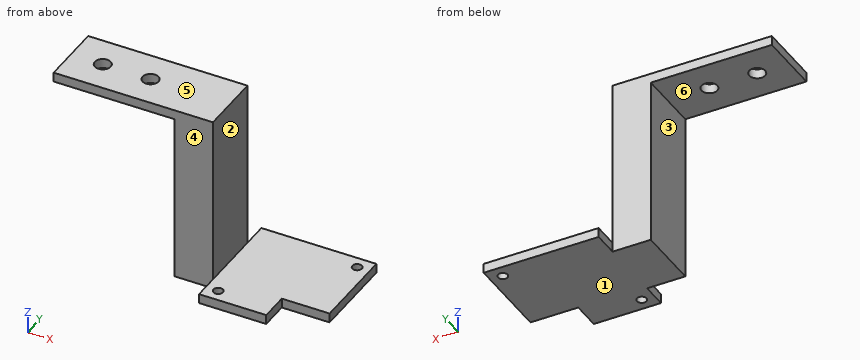
from build123d import *

# Parameters (mm, degrees)
SKETCH_1_W          = 36.1
SKETCH_1_H          = 36.1
EXTRUDE_1_DEPTH     = 3
SKETCH_2_R          = 1.5
CUT_EXTRUDE_1_DEPTH = 3
SKETCH_3_W          = 15
SKETCH_3_H          = 9
CUT_EXTRUDE_2_DEPTH = 3
SKETCH_4_W          = 12
SKETCH_4_H          = 10
EXTRUDE_2_DEPTH     = 3
SKETCH_5_W          = 12
SKETCH_5_H          = 20
EXTRUDE_3_DEPTH     = 50
SKETCH_7_W          = 50
SKETCH_7_H          = 20
EXTRUDE_4_DEPTH     = 3
SKETCH_9_R          = 2.5
CUT_EXTRUDE_4_DEPTH = 3


with BuildPart() as part:
    # 草图1 → 凸台-拉伸1 (new body)
    with BuildSketch(Plane.XY):
        Rectangle(SKETCH_1_W, SKETCH_1_H)
    extrude(amount=EXTRUDE_1_DEPTH)

    # 草图2 → 切除-拉伸1 (cut)
    with BuildSketch(Plane.XY.offset(3)):
        with Locations((14.142135624, 14.142135624)):
            Circle(SKETCH_2_R)
        with Locations(Location((-14.142135624, -14.142135624, 0), (0, 0, 180))):
            Circle(SKETCH_2_R)
    extrude(amount=-CUT_EXTRUDE_1_DEPTH, mode=Mode.SUBTRACT)

    # 草图3 → 切除-拉伸2 (cut)
    with BuildSketch(Plane.XY.offset(3)):
        with Locations((10.55, -13.55)):
            Rectangle(SKETCH_3_W, SKETCH_3_H)
    extrude(amount=-CUT_EXTRUDE_2_DEPTH, mode=Mode.SUBTRACT)

    # 草图4 → 凸台-拉伸2 (add)
    with BuildSketch(Plane.XY.offset(3)):
        with Locations((-24.05, 5)):
            Rectangle(SKETCH_4_W, SKETCH_4_H)
        with Locations((-24.05, -5)):
            Rectangle(SKETCH_4_W, SKETCH_4_H)
    extrude(amount=-EXTRUDE_2_DEPTH)

    # 草图5 → 凸台-拉伸3 (add)
    with BuildSketch(Plane.XY.offset(3)):
        with Locations((-24.05, 0)):
            Rectangle(SKETCH_5_W, SKETCH_5_H)
    extrude(amount=EXTRUDE_3_DEPTH)

    # 草图7 → 凸台-拉伸4 (add)
    with BuildSketch(Plane.XY.offset(53)):
        with Locations((-43.05, 0)):
            Rectangle(SKETCH_7_W, SKETCH_7_H)
    extrude(amount=EXTRUDE_4_DEPTH)

    # 草图9 → 切除-拉伸4 (cut)
    with BuildSketch(Plane.XY.offset(56)):
        with Locations((-58.05, 0)):
            Circle(SKETCH_9_R)
        with Locations((-43.05, 0)):
            Circle(SKETCH_9_R)
    extrude(amount=-CUT_EXTRUDE_4_DEPTH, mode=Mode.SUBTRACT)


solid = part.part
Verification items for the finished model (mm, model axes). Face numbers are marked on the shaded views. A direction names the side the tool comes from. Give positions to 0.01 mm unless a question says otherwise; leave off trailing zeros. Write each loop counter-clockwise with the first axis right and the second up, starting at its lowest first coordinate (ties: lowest second). Pieces come first, ordered by that corner, then holes. Notation, with made-up numbers: (76, 20) - (130, 20) arc R21 cw to (130, 48) - close; hole circle Ø8 at (51.25, 9.25). An arc over 180 degrees is marked (long way). Answer as CSV lines item,"result". Start each with the question number.
1. Depth check by flat-ended pin: pin 1 (4 mm diameter, centred on x = 14.14, y = 14.14, fed in from +Z); pin 2 (2.5 mm diameter, centred on y = 15.5, z = 1, fed in from -X); pin 3 (2.5 mm diameter, centred on y = -15.5, z = 1.5, fed in from +X). Enter the tip coordinate at first touch or a pass-through.
2. Draft check along Z on the marked faces 4, 5 and 6. Enter one of: pulls with the +Z half, pulls with the -Z half, needs draft (parallel to the pull), parting line crosses it, or undercut.
3. Set-up check for the marked faces 1, 2 and 3: record each of +Z, -Z, +X, -X, +Y, -Y from which the full face is reachable in a straight line by a thin tool's end or side.
4. Sectioned sample at A-A (y = 0). Record the boundary of the cut face in (x, z).
5. Thickness scan on line 1 (Y direction, x = -58.05, z = 54.55); line 2 (Z direction, x = -12, y = 16); line 3 (Z direction, x = -38.5, y = 1). Record the ranges inside material, lowest first.
6. Sectioned sample at B-B (x = -58.05). Record the boundary of the cut face in (y, z), then the cut area to 3 significant figures.
7. Sectioned sample at C-C (z = 31). Record the boundary of the cut face in (x, y).
8. Sectioned sample at D-D (x = -23). Record the boundary of the cut face in (y, z), then the cut area to 3 significant figures.
Derived:
1,pin 1,"z = 3"
1,pin 2,"x = -18.05"
1,pin 3,"x = 3.05"
2,face 4,"needs draft"
2,face 5,"pulls with the +Z half"
2,face 6,"pulls with the -Z half"
3,face 1,"-Z, +X, -X, +Y, -Y"
3,face 2,"+Z, +X, +Y, -Y"
3,face 3,"-Z, -X, +Y, -Y"
4,outline,"(-68.05, 53) - (-60.55, 53) - (-60.55, 56) - (-68.05, 56) - close; (-55.55, 53) - (-45.55, 53) - (-45.55, 56) - (-55.55, 56) - close; (-40.55, 53) - (-30.05, 53) - (-30.05, 0) - (18.05, 0) - (18.05, 3) - (-18.05, 3) - (-18.05, 56) - (-40.55, 56) - close"
5,line 1,"-10 to -2.5, 2.5 to 10"
5,line 2,"0 to 3"
5,line 3,"53 to 56"
6,outline,"(-10, 53) - (-2.5, 53) - (-2.5, 56) - (-10, 56) - close; (2.5, 53) - (10, 53) - (10, 56) - (2.5, 56) - close"
6,area,"45.0 mm²"
7,outline,"(-30.05, -10) - (-18.05, -10) - (-18.05, 10) - (-30.05, 10) - close"
8,outline,"(-10, 0) - (10, 0) - (10, 56) - (-10, 56) - close"
8,area,"1,120 mm²"
